Input: part model. Units: mm. Frame: model coordinates. Round coordinates to 2 decimals unless told otherwise and drop trailing zeros. Write each loop counter-clockwise with the first axis right and the second up, starting at its lowest first coordinate (ties: lowest second). Pieces come first, ordered by that corner, then holes. Notation, with made-up numbers: (22.5, -32.5) -> (57.5, -32.5) arc R23 ccw to (57.5, -0.5) -> close; hole circle Ø3 at (44, -12). An arc over 180 degrees is marked (long way). Use CSV: the item, a comma, the result in double quotes.
```python
from build123d import *

# Parameters (mm, degrees)
F0_W     = 1257.3
F0_H     = 88.9
F1_DEPTH = 19.05
F3_DEPTH = 127
F5_DEPTH = 127


with BuildPart() as f1:
    # F0 (on Front) → F1 (new body)
    with BuildSketch(Plane.XZ):
        with Locations((-628.65, 44.45)):
            Rectangle(F0_W, F0_H)
    extrude(amount=F1_DEPTH)

    # F2 (on face) → F3 (cut)
    with BuildSketch(Plane(origin=(0, 0, 0), x_dir=(1, 0, 0), z_dir=(0, 0, -1))):
        Polygon((-1257.3, 19.05), (-1257.3, 0), (-1238.25, 19.05), align=None)
    extrude(amount=-F3_DEPTH, mode=Mode.SUBTRACT)

    # F4 (on face) → F5 (cut)
    with BuildSketch(Plane(origin=(0, 0, 0), x_dir=(1, 0, 0), z_dir=(0, 0, -1))):
        Polygon((-19.05, 19.05), (0, 0), (0, 19.05), align=None)
    extrude(amount=-F5_DEPTH, mode=Mode.SUBTRACT)


solid = f1.part
```
Item 1: Line query: line 1 (X direction, y = -12.75, z = 34); line 2 (X direction, y = -7, z = 80). Output: solid intervals per line, ascending.
Worked answers:
line 1,"x = -1244.55 to -12.75"
line 2,"x = -1250.3 to -7"
Item 2: Section query B-B on y = -9.5. Return the cut outline in (x, z).
Worked answers:
outline,"(-1247.8, 0) -> (-9.5, 0) -> (-9.5, 88.9) -> (-1247.8, 88.9) -> close"
Item 3: First-contact query: pin 1 Ø6 at (x, y) = (-1103, -3.5) entering from -Z. Flat tip, straight axial feed; report the tip coordinate or a pass-through.
Worked answers:
pin 1,"stops at z = 0"
Item 4: Section query A-A on z = 25.5. Return the cut outline in (x, y).
Worked answers:
outline,"(-1257.3, 0) -> (-1238.25, -19.05) -> (-19.05, -19.05) -> (0, 0) -> close"
